from build123d import *

# Parameters (mm, degrees)
SKETCH_1_W                       = 5
SKETCH_1_H                       = 7
SM_BASE_FLANGE_1_DEPTH           = 0.8
SM_EDGE_FLANGE_1_STRIP_W         = 4.6732
SM_EDGE_FLANGE_1_STRIP_H         = 0.8
SM_EDGE_FLANGE_1_STRIP_CUT_DEPTH = 5
SM_EDGE_FLANGE_1_DEPTH           = 5
SKETCH_7_R                       = 1.25
CUT_EXTRUDE_1_DEPTH              = 10
SKETCH_8_W                       = 1.1
SKETCH_8_H                       = 7.5
CUT_EXTRUDE_2_DEPTH              = 10
SKETCH_9_R                       = 0.6
CUT_EXTRUDE_3_DEPTH              = 10
CHAMFER_1_SIZE                   = 0.8


# Sheet-metal steps are written as plain solids
with BuildPart() as part:
    # Sketch 1 → 基体-法兰1 (new body)
    with BuildSketch(Plane.XY):
        Rectangle(SKETCH_1_W, SKETCH_1_H)
    extrude(amount=-SM_BASE_FLANGE_1_DEPTH)

    # 边线-法兰1 strip (across the edge) → 边线-法兰1 strip cut (cut)
    with BuildSketch(Plane(origin=(-2.5, 3.5, -0.8), x_dir=(0, -1, 0), z_dir=(1, 0, 0))):
        with Locations((-0.8, -0.4)):
            Rectangle(SM_EDGE_FLANGE_1_STRIP_W, SM_EDGE_FLANGE_1_STRIP_H)
    extrude(amount=SM_EDGE_FLANGE_1_STRIP_CUT_DEPTH, mode=Mode.SUBTRACT)

    # 边线-法兰1 section (across the edge) → 边线-法兰1 (add)
    with BuildSketch(Plane(origin=(-2.5, 3.5, -0.8), x_dir=(0, -1, 0), z_dir=(1, 0, 0))):
        with BuildLine():
            Line((0, 0.7366), (0, 8.7))
            Line((0, 8.7), (0.8, 8.7))
            Line((0.8, 8.7), (0.8, 0.7366))
            ThreePointArc((0.8, 0.7366), (1.015745145, 0.215745145), (1.5366, 0))
            Line((1.5366, 0), (1.5366, -0.8))
            ThreePointArc((1.5366, -0.8), (0.45005972, -0.34994028), (0, 0.7366))
        make_face()
    extrude(amount=SM_EDGE_FLANGE_1_DEPTH)

    # 草图7 → 切除-拉伸1 (cut)
    with BuildSketch(Plane(origin=(0, 0, -0.8), x_dir=(-1, 0, 0), z_dir=(0, 0, -1))):
        with Locations((0, -0.7683)):
            Circle(SKETCH_7_R)
    extrude(amount=-CUT_EXTRUDE_1_DEPTH, mode=Mode.SUBTRACT)

    # 草图8 → 切除-拉伸2 (cut)
    with BuildSketch(Plane(origin=(0, 3.5, 0), x_dir=(1, 0, 0), z_dir=(0, 1, 0))):
        with Locations((1.95, 5.75)):
            Rectangle(SKETCH_8_W, SKETCH_8_H)
        with Locations((-1.95, 5.75)):
            Rectangle(SKETCH_8_W, SKETCH_8_H)
    extrude(amount=-CUT_EXTRUDE_2_DEPTH, mode=Mode.SUBTRACT)

    # 草图9 → 切除-拉伸3 (cut)
    with BuildSketch(Plane(origin=(0, 3.5, 0), x_dir=(1, 0, 0), z_dir=(0, 1, 0))):
        with Locations(Location((0, 7.951292253, 0), (0, 0, 270))):
            Circle(SKETCH_9_R)
    extrude(amount=-CUT_EXTRUDE_3_DEPTH, mode=Mode.SUBTRACT)

    # 倒角1
    chamfer_1_edges = [part.edges().sort_by_distance(p)[0] for p in [
        (-1.4, 3.1, -9.5),
        (1.4, 3.1, -9.5),
    ]]
    chamfer(chamfer_1_edges, length=CHAMFER_1_SIZE)


solid = part.part
Build history of the part. All positions in model axes, mm. A direction names the side the tool comes from. Coordinates: 2 decimals unless noted, no trailing zeros. Order: outer loops, then holes, each group sorted by start corner. A loop starts at its lowest first (then second) coordinate and runs counter-clockwise, first axis right, second up. Notation, with made-up numbers: (58, 9) - (83, 9) arc R16 cw to (83, 19) - close; hole circle Ø7 at (-17, 83). An arc over 180 degrees is marked (long way). Put each result on its own line as item: value.
1. Saw through at D-D (x = 1.05). Write the cut outline in (y, z).
Answer sheet:
outline: (-3.5, -0.8) - (-1.45, -0.8) - (-1.45, 0) - (-3.5, 0) - close; (-0.09, -0.8) - (1.96, -0.8) arc R0.74 cw to (2.7, -1.54) - (2.7, -9.05) - (3.5, -9.05) - (3.5, -1.54) arc R1.54 ccw to (1.96, 0) - (-0.09, 0) - close
2. Tool access for faces 1 (the face through (0.27, -1.99, -0.41)), 2 (the face through (-0.6, 0.5, -0.8)): list every direction of +Z, -Z, +X, -X, +Y, -Y with a clear straight run to the whole face (end or side of a thin tool).
Answer sheet:
face 1: +Z, -Z
face 2: -Z, +X, -X, -Y
3. Drop flat-ended pins along their axis: P1, Ø1.4, axis at x = 0, z = -7.95, coming from the -Y side; P2, Ø1.5, axis at x = 0.5, y = -1, coming from the -Z side; P3, Ø3, axis at y = 2, z = -5.5, coming from the -X side. Give the stop position or say it passes through.
Answer sheet:
P1: stops at y = 2.7
P2: stops at z = -0.8
P3: stops at x = -1.4
4. Saw through at B-B (z = -8). Write the cut outline in (x, y), and give its area (3 significant figures).
Answer sheet:
outline: (-1.4, 2.7) - (-0.6, 2.7) - (-0.6, 3.5) - (-1.4, 3.5) - close; (0.6, 2.7) - (1.4, 2.7) - (1.4, 3.5) - (0.6, 3.5) - close
area: 1.28 mm^2
5. Probe line 1 along Z through (x, y) = (-2.3, -0.5); line 2 along Y through (x, z) = (-0.9, -3.5); line 3 along X through (y, z) = (2.75, -7.5). List the from-to ranges inside material, lowest first. Write a range as [from, to].
Answer sheet:
line 1: z = [-0.8, 0]
line 2: y = [2.7, 3.5]
line 3: x = [-1.4, -0.4], [0.4, 1.4]
6. Saw through at A-A (x = 0). Write the cut outline in (y, z), and give its area (3 significant figures).
Answer sheet:
outline: (-3.5, -0.8) - (-2.02, -0.8) - (-2.02, 0) - (-3.5, 0) - close; (0.48, -0.8) - (1.96, -0.8) arc R0.74 cw to (2.7, -1.54) - (2.7, -7.35) - (3.5, -7.35) - (3.5, -1.54) arc R1.54 ccw to (1.96, 0) - (0.48, 0) - close; (2.7, -9.5) - (3.5, -9.5) - (3.5, -8.55) - (2.7, -8.55) - close
area: 9.21 mm^2
7. Saw through at C-C (y = -1.5). Write the cut outline in (x, z), and give its area (3 significant figures).
Answer sheet:
outline: (-2.5, -0.8) - (-1.01, -0.8) - (-1.01, 0) - (-2.5, 0) - close; (1.01, -0.8) - (2.5, -0.8) - (2.5, 0) - (1.01, 0) - close
area: 2.38 mm^2
8. Pull direction Z, two halves, no side cores. Call faces 3 (the face through (-1, 3.1, -9.1)), 4 (the face through (-2.5, 0, -0.6)), 5 (the face through (0.03, 3.11, -8.55)): pulls with the +Z half, pulls with the -Z half, needs draft (parallel to the pull), parting line crosses it, or undercut.
Answer sheet:
face 3: pulls with the -Z half
face 4: needs draft
face 5: undercut
